Source: CAD feature listing. Evaluate the final solid. Frame: model axes, mm. A direction names the side the tool comes from. Give positions to 0.01 mm unless a question says otherwise; leave off trailing zeros. Loops run counter-clockwise (first coordinate to the right, second up) from the corner with the lowest first, then second, coordinate; pieces in that order, holes last. Notation, with made-up numbers: (76, -17) -> (101, -17) arc R30 cw to (101, 10) -> close; hole circle Ø11 at (0.25, 75). An arc over 180 degrees is marked (long way). Return JSON: item names as keys, results as strings. Group by question number.
(1) Pin query (flat end, axial travel): pin 1 (15.5 mm diameter, centred on x = 519.5, y = 95.5, fed in from +Z); pin 2 (6 mm diameter, centred on x = 506, z = -63, fed in from +Y); pin 3 (8 mm diameter, centred on x = 551.5, z = -72.5, fed in from +Y). Return the tip coordinate at first contact, or that it passes through.
(2) Cut plane B-B on x = 513.5. Return loops of the section in (y, z), then the cut area to 3 significant figures.
(3) Cut plane A-A on z = -42.5. Return loops of the section in (x, y).
(4) Access query for faces 1 (the face through (530.35, 93.65, -16.51)), 2 (the face through (502, 103, -114.3)), 3 (the face through (506.304, 101.837, -16.515)). Directions: +Z, -Z, +X, -X, +Y, -Y. A direction counts if a zero-diameter tool reaches every point of the face in a straight line with its end or side. Return the directions, or none.
(5) Ray query, line 1 (Y direction, x = 485.5, z = -28); line 2 (Y direction, x = 559, z = -34.5). Return the intervals inside material, ascending. Write a range as from..to.
```python
from build123d import *

# Parameters (mm, degrees)
BOSS_EXTRUDE2_DEPTH = 114.3
CUT_EXTRUDE1_REACH  = 541.354
SKETCH2_W           = 25.4
SKETCH2_H           = 40.79687197


with BuildPart() as part:
    # Sketch1 → Boss-Extrude2 (new body)
    with BuildSketch(Plane.XY):
        Polygon((581.808782497, 79.428009058), (425.537875129, 132.65163668), (423.490637562, 126.640703446), (579.76154493, 73.417075823), align=None)
    extrude(amount=-BOSS_EXTRUDE2_DEPTH)

    # Sketch2 → Cut-Extrude1 (cut, up to next)
    with BuildSketch(Plane(origin=(84.714294761, 248.731255285, 0), x_dir=(0.9466036589314765, -0.3223996167763558, 0), z_dir=(0.32239961677635576, 0.9466036589314764, 0)), mode=Mode.PRIVATE) as cut_extrude1_sk1:
        with Locations((459.137216198, 13.100047516)):
            Rectangle(SKETCH2_W, SKETCH2_H)
    cut_extrude1_tool1 = extrude(cut_extrude1_sk1.sketch, amount=-CUT_EXTRUDE1_REACH, mode=Mode.PRIVATE) & part.part
    add(cut_extrude1_tool1.solids().sort_by_distance((519.335264, 100.705593, -13.100048))[0], mode=Mode.SUBTRACT)


solid = part.part
```
Answers:
{
 "1": {"pin 1": "z = -33.5", "pin 2": "y = 106.27", "pin 3": "y = 91.11"},
 "2": {"outline": "(95.98, -114.3) -> (102.69, -114.3) -> (102.69, -33.5) -> (95.98, -33.5) -> close", "area": "542 mm²"},
 "3": {"outline": "(423.49, 126.64) -> (579.76, 73.42) -> (581.81, 79.43) -> (425.54, 132.65) -> close"},
 "4": {"face 1": "+Z, -X, +Y", "face 2": "-Z, +X, -X, +Y, -Y", "face 3": "+Z, +X, -Y"},
 "5": {"line 1": "105.52..112.23", "line 2": "80.49..87.2"}
}
